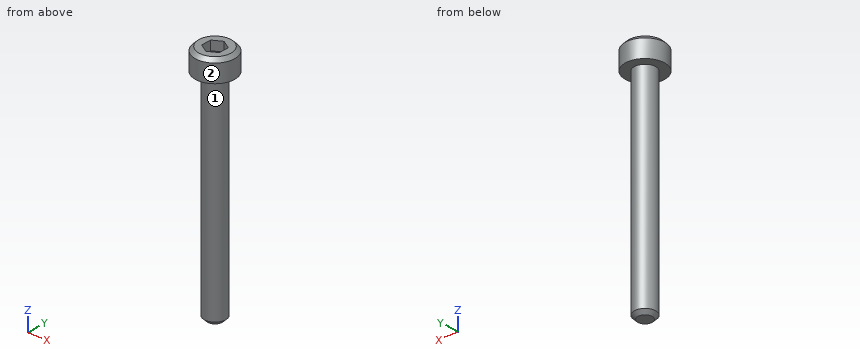
Autodesk Inventor part; units mm, degrees
ref_plane "YZ Plane" through (0, 0, 0) normal (1, 0, 0) x (0, 1, 0)
ref_plane "XZ Plane" through (0, 0, 0) normal (0, 1, 0) x (-1, 0, 0)
ref_plane "XY Plane" through (0, 0, 0) normal (0, 0, 1) x (1, 0, 0)
sketch "Sketch1" plane through (0, 0, 0) normal (0, 0, 1) x (1, 0, 0)
  circle A0 centre (0, 0) radius 1.5
  dimension "Diameter" = 3
extrude "Extrusion1" add sketch "Sketch1" along normal blind 30
sketch "Sketch2" plane through (0, 0, 30) normal (0, 0, 1) x (1, 0, 0)
  circle A0 centre (0, 0) radius 1.5
  circle A1 centre (0, 0) radius 2.75
  dimension "Kopdiameter" = 5.5
extrude "Extrusion2" add sketch "Sketch2" along normal blind 3 contours A0 | A1
sketch "Sketch3" plane through (0, 0, 33) normal (0, 0, 1) x (1, 0, 0)
  circle A0 centre (0, 0) radius 2.75
  circle A1 centre (0, 0) radius 1.4434 construction
  line L0 (0, 1.4434) -> (1.25, 0.7217)
  line L1 (1.25, -0.7217) -> (1.25, 0.7217)
  line L2 (0, 1.4434) -> (-1.25, 0.7217)
  line L3 (-1.25, -0.7217) -> (-1.25, 0.7217)
  line L4 (-1.25, -0.7217) -> (0, -1.4434)
  line L5 (1.25, -0.7217) -> (0, -1.4434)
  dimension "Binnenzeskant" = 2.5
extrude "Extrusion3" cut sketch "Sketch3" against normal blind 1.3 contours L0 L1 L5 L4 L3 L2
thread "Thread1"
chamfer "Chaflán2" distance 0.5 angle 45 2 edges at (-2.75, 0, 33) (-1.5, 0, 0)
equation "\"d9\" = Draadlengte"
equation "\"Draadlengte\" = 24.75"
equation "\"Sizes\" = Diameter"
equation "\"Schroefdraad\" = Sizes"
properties part number "tornillo allen m3x30" material "Grade 8.8"
For this review, take the finished solid that the model builds, in its own axes (mm). Face numbers are marked on the shaded views. A direction names the side the tool comes from. Give positions to 0.01 mm unless a question says otherwise; leave off trailing zeros. Loops run counter-clockwise (first coordinate to the right, second up) from the corner with the lowest first, then second, coordinate; pieces in that order, holes last. Notation, with made-up numbers: M 22,24 L 53,24 A34 ccw 53,62 Z; hole C 75,-15.5 d5. An arc over 180 degrees is marked long. One line per item, written item: value. Start each with the question number.
Q1. Clearance check with flat-ended pins moving along their axes: pin 1 Ø2 at (y, z) = (0.5, 28) entering from +X; pin 2 Ø0.7 at (y, z) = (0.5, 32) entering from +X; pin 3 Ø3 at (y, z) = (1.5, 6) entering from -X. State where each tip first meets the part, or that it passes through.
Q2. Add section A-A (y = 0). Give the boundary of the cut face in (x, z), and give its area (3 significant figures).
Q3. Add section B-B (z = 6). Give the boundary of the cut face in (x, y), and give its area (3 significant figures).
Q4. For L1, parallel to Z at x = 0.95, y = -1.9; L2, parallel to Z at x = -0.1, y = 0.75; L3, parallel to X at y = -0.65, z = 5.5, list the stretches that pass through material, from the lowest coordinate up.
Q5. Machinability: for the marked faces 1 and 2, which of the approach directions +Z, -Z, +X, -X, +Y, -Y give a long, thin tool a straight path to every point of the face, cutting with its end or side? Answer none if there is none.
Reply:
1. pin 1: x = 1.5
1. pin 2: x = 2.75
1. pin 3: x = -1.5
2. outline: M -2.75,30 L -1.5,30 L -1.5,0.5 L -1,0 L 1,0 L 1.5,0.5 L 1.5,30 L 2.75,30 L 2.75,32.5 L 2.25,33 L 1.25,33 L 1.25,31.7 L -1.25,31.7 L -1.25,33 L -2.25,33 L -2.75,32.5 Z
2. area: 103 mm²
3. outline: C 0,0 d3
3. area: 7.07 mm²
4. L1: 30 to 33
4. L2: 0 to 31.7
4. L3: -1.35 to 1.35
5. face 1: -Z
5. face 2: +Z, -Z
